Input: part model. Units: mm. Frame: model coordinates. Coordinates: 2 decimals unless noted, no trailing zeros. Loops run counter-clockwise (first coordinate to the right, second up) from the corner with the lowest first, then second, coordinate; pieces in that order, holes last.
```python
from build123d import *

# Parameters (mm, degrees)
BOSS_EXTRUDE1_DEPTH = 6
SKETCH2_R           = 2.8
SKETCH2_R_2         = 5
SKETCH2_R_3         = 1.43
CUT_EXTRUDE1_DEPTH  = 7


with BuildPart() as part:
    # Sketch1 → Boss-Extrude1 (new body)
    with BuildSketch(Plane.XY):
        Polygon((0, 200), (0, 5), (-5, 0), (-118, 0), (-118, 25), (-60, 25), (-60, 200), (-55, 205), (-5, 205), align=None)
    extrude(amount=BOSS_EXTRUDE1_DEPTH)

    # Sketch2 → Cut-Extrude1 (cut, through all)
    with BuildSketch(Plane.XY.offset(6)):
        with Locations((-108, 19)):
            Circle(SKETCH2_R)
        with Locations((-108, 5)):
            Circle(SKETCH2_R)
        with Locations((-30, 170)):
            Circle(SKETCH2_R_2)
        with Locations((-19.6, 163.9955572)):
            Circle(SKETCH2_R_3)
        with Locations((-40.4, 163.9955572)):
            Circle(SKETCH2_R_3)
        with Locations((-30, 182.008885599)):
            Circle(SKETCH2_R_3)
    extrude(amount=-CUT_EXTRUDE1_DEPTH, mode=Mode.SUBTRACT)


solid = part.part
```
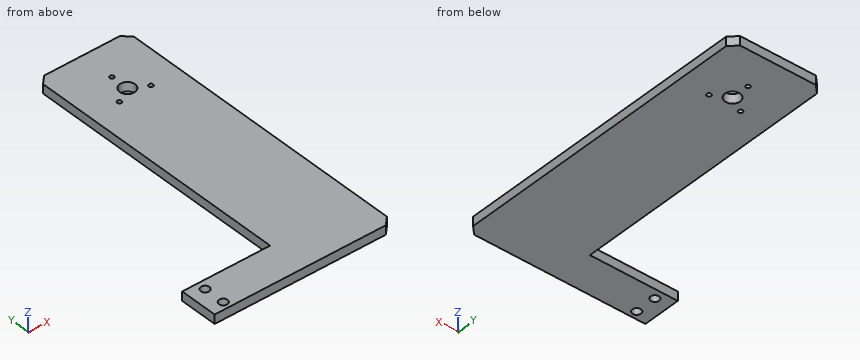
Item 1: Section query A-A (y = 19). Output: boundary loops of the cut face in (x, z), then the cut area to 3 significant figures.
Result:
outline: (-118, 0) - (-110.8, 0) - (-110.8, 6) - (-118, 6) - close; (-105.2, 0) - (0, 0) - (0, 6) - (-105.2, 6) - close
area: 674 mm2
Item 2: Section query D-D (z = 4.5). Output: boundary loops of the cut face in (x, y), then the cut area to 3 significant figures.
Result:
outline: (-118, 0) - (-5, 0) - (0, 5) - (0, 200) - (-5, 205) - (-55, 205) - (-60, 200) - (-60, 25) - (-118, 25) - close; hole circle Ø5.6 at (-108, 5); hole circle Ø5.6 at (-108, 19); hole circle Ø2.86 at (-40.4, 164); hole circle Ø10 at (-30, 170); hole circle Ø2.86 at (-30, 182.01); hole circle Ø2.86 at (-19.6, 164)
area: 13,600 mm2
Item 3: Section query C-C (y = 170). Output: boundary loops of the cut face in (x, z).
Result:
outline: (-60, 0) - (-35, 0) - (-35, 6) - (-60, 6) - close; (-25, 0) - (0, 0) - (0, 6) - (-25, 6) - close
Item 4: Line query: L1, parallel to Y at x = -30, z = 3.3; L2, parallel to Y at x = -108, z = 3.05; L3, parallel to Y at x = -101, z = 1.2. Output: solid intervals per line, ascending.
Result:
L1: y = 0 to 165, 175 to 180.58, 183.44 to 205
L2: y = 0 to 2.2, 7.8 to 16.2, 21.8 to 25
L3: y = 0 to 25
Item 5: Section query B-B (x = -108). Output: boundary loops of the cut face in (y, z).
Result:
outline: (0, 0) - (2.2, 0) - (2.2, 6) - (0, 6) - close; (7.8, 0) - (16.2, 0) - (16.2, 6) - (7.8, 6) - close; (21.8, 0) - (25, 0) - (25, 6) - (21.8, 6) - close
Item 6: Contact query for flat-ended pins moving along their axis: P1, Ø3, axis at y = 117.5, z = 2.5, coming from the -X side; P2, Ø4.5, axis at x = -108, y = 19, coming from the +Z side. Output: stop coordinate, or through.
Result:
P1: stops at x = -60
P2: passes through
